Part model, mm, in its own coordinate system. A direction names the side the tool comes from. Give positions to 0.01 mm unless a question says otherwise; leave off trailing zeros. Write each loop counter-clockwise with the first axis right and the second up, starting at its lowest first coordinate (ties: lowest second). Pieces come first, ordered by that corner, then holes. Notation, with made-up numbers: M -16.75,57.5 L -3.75,57.5 A13 ccw -3.75,74.5 Z; hole C -2,-32 d4. An arc over 180 degrees is marked long. Write item = value, one per line. Start each with the question number.
Autodesk Inventor part; units mm, degrees
ref_plane "YZ Plane" through (0, 0, 0) normal (1, 0, 0) x (0, 1, 0)
ref_plane "XZ Plane" through (0, 0, 0) normal (0, 1, 0) x (-1, 0, 0)
ref_plane "XY Plane" through (0, 0, 0) normal (0, 0, 1) x (1, 0, 0)
sketch "Sketch1" plane through (0, 0, 0) normal (0, 0, 1) x (1, 0, 0)
  line L0 (-4.4697, -5.5303) -> (4.4697, 5.5303) construction
  line L1 (5.5303, 4.4697) -> (-5, -4.0411) construction
  line L2 (4.4697, -5.5303) -> (-4.4697, 5.5303) construction
  line L3 (-5.5303, 4.4697) -> (5.5303, -4.4697) construction
  line L4 (-5, -5) -> (-5, -3.9393)
  line L5 (-5, 3.9393) -> (-5, 5)
  line L6 (5, 5) -> (5, 3.9393)
  line L7 (5, -3.9393) -> (5, -5)
  line L8 (-5, 5) -> (-3.9393, 5)
  line L9 (3.9393, 5) -> (5, 5)
  line L10 (5, -5) -> (3.9393, -5)
  line L11 (-3.9393, -5) -> (-5, -5)
  line L12 (-2.6893, 3.75) -> (-0.4393, 1.5)
  line L13 (2.6893, 3.75) -> (0.4393, 1.5)
  line L14 (-1.5, -0.4393) -> (-3.75, -2.6893)
  line L15 (-1.5, 0.4393) -> (-3.75, 2.6893)
  line L16 (2.6893, -3.75) -> (0.4393, -1.5)
  line L17 (-2.6893, -3.75) -> (-0.4393, -1.5)
  line L18 (1.5, 0.4393) -> (3.75, 2.6893)
  line L19 (1.5, -0.4393) -> (3.75, -2.6893)
  line L20 (5, -5) -> (-5, 5) construction
  line L21 (-5, -5) -> (5, 5) construction
  line L22 (3.75, -3.75) -> (-3.75, 3.75) construction
  line L23 (-3.75, -3.75) -> (3.75, 3.75) construction
  line L24 (1.5, -5) -> (-1.5, 5) construction
  line L25 (-1.5, -5) -> (1.5, 5) construction
  line L26 (5, -1.5) -> (-5, 1.5) construction
  line L27 (-5, -1.5) -> (5, 1.5) construction
  line L28 (-5, 1.5) -> (-3.75, 1.5)
  line L29 (-3.75, -1.5) -> (-5, -1.5)
  line L30 (-3.75, -2.6893) -> (-3.75, -1.5)
  line L31 (-3.75, 1.5) -> (-3.75, 2.6893)
  line L32 (-5, -5) -> (-5, -1.5)
  line L33 (-5, 1.5) -> (-5, 5)
  line L34 (-5, 5) -> (-1.5, 5)
  line L35 (1.5, 5) -> (5, 5)
  line L36 (-1.5, 3.75) -> (-1.5, 5)
  line L37 (-2.6893, 3.75) -> (-1.5, 3.75)
  line L38 (1.5, 3.75) -> (2.6893, 3.75)
  line L39 (1.5, 5) -> (1.5, 3.75)
  line L40 (3.75, 1.5) -> (5, 1.5)
  line L41 (3.75, 2.6893) -> (3.75, 1.5)
  line L42 (3.75, -1.5) -> (3.75, -2.6893)
  line L43 (5, 5) -> (5, 1.5)
  line L44 (5, -1.5) -> (5, -5)
  line L45 (5, -1.5) -> (3.75, -1.5)
  line L46 (-0.45, 1.5) -> (0.45, 1.5)
  line L47 (-1.5, -5) -> (-1.5, -3.75)
  line L48 (-1.5, -0.45) -> (-1.5, 0.45)
  line L49 (1.5, 0.45) -> (1.5, -0.45)
  line L50 (2.6893, -3.75) -> (1.5, -3.75)
  line L51 (5, -5) -> (1.5, -5)
  line L52 (-1.5, -5) -> (-5, -5)
  line L53 (1.5, -3.75) -> (1.5, -5)
  line L54 (0.45, -1.5) -> (-0.45, -1.5)
  line L55 (-1.5, -3.75) -> (-2.6893, -3.75)
  point P0 (0, 0)
  point P1 (0, 0)
  dimension "d0" = 10
  dimension "d7" = 1.5
  dimension "d8" = 1.5
  dimension "d9" = 7.5
  dimension "d10" = 7.5
  dimension "d11" = 10
  dimension "d12" = 3
  dimension "d13" = 3
extrude "Extrusion1" add sketch "Sketch1" along normal blind 40
equation "\"d8\" = d7"
equation "\"d10\" = d9"
equation "\"d11\" = d0"
equation "\"d4\" = 0.5 * d0"
equation "\"d5\" = 0.5 * d0"
equation "\"d6\" = 0.5 * d0"
properties part number "maker-beam-40x10x10mm"
Q1. Slice it at B-B (y = 0). Give the cut face in (x, z), and give its area (3 significant figures).
Q2. Drop flat-ended pins along their axis: P1, Ø1, axis at x = 3, y = 0, coming from the +Z side; P2, Ø0.7, axis at y = 0, z = 25.5, coming from the -X side; P3, Ø1, axis at x = 0, z = 17, coming from the +Y side. Give the stop position or say it passes through.
Q3. Tool access for faces 1 (the face through (3, -5, 20)), 2 (the face through (4, -1.5, 20)), 3 (the face through (2.61, 1.55, 19.72)), 4 (the face through (3, 5, 20)), 5 (the face through (0, 1.5, 20)): list every direction of +Z, -Z, +X, -X, +Y, -Y with a clear straight run to the whole face (end or side of a thin tool).
Q4. Two-plate mould, pull along Y, no slides. Class faces 6 (the face through (0, -1.5, 20)), 7 (the face through (1.5, 4, 20)), 8 (the face through (-2.61, -1.55, 19.72)): +Y half, -Y half, draft (parallel to the pull), parting line (faces both ways), or undercut.
Q5. Probe line 1 along X through (y, z) = (2, 2); line 2 along X through (y, z) = (2.5, 32); line 3 along X through (y, z) = (2.75, 12.5). List the from-to ranges inside material, lowest first.
Q6. Slice it at A-A (y = -3.25). Give the cut face in (x, z), and give its area (3 significant figures).
Working result:
q1.outline = M -1.5,0 L 1.5,0 L 1.5,40 L -1.5,40 Z
q1.area = 120 mm2
q2.P1 = through
q2.P2 = -1.5
q2.P3 = 1.56
q3.face_1 = +Z, -Z, +X, -X, -Y
q3.face_2 = +Z, -Z, +X
q3.face_3 = +Z, -Z
q3.face_4 = +Z, -Z, +X, -X, +Y
q3.face_5 = +Z, -Z, +Y
q4.face_6 = -Y half
q4.face_7 = draft
q4.face_8 = undercut
q5.line_1 = -5 to -3.75, -3.06 to -0.94, 0.94 to 3.06, 3.75 to 5
q5.line_2 = -5 to -3.75, -3.56 to -1.44, 1.44 to 3.56, 3.75 to 5
q5.line_3 = -5 to -1.69, 1.69 to 5
q6.outline = M -5,0 L -2.19,0 L -2.19,40 L -5,40 Z; M 2.19,0 L 5,0 L 5,40 L 2.19,40 Z
q6.area = 225 mm2
